Build history of the part. All positions in model axes, mm. A direction names the side the tool comes from. Round coordinates to 2 decimals unless told otherwise and drop trailing zeros. Write each loop counter-clockwise with the first axis right and the second up, starting at its lowest first coordinate (ties: lowest second). Pieces come first, ordered by that corner, then holes. Notation, with made-up numbers: M 25.25,32.5 L 69.25,32.5 A6 ccw 69.25,36.5 Z; hole C 59,84 d9. An arc over 180 degrees is marked long. Write item = value, one per line.
from build123d import *

# Parameters (mm, degrees)
F0_W     = 1016
F0_H     = 381
F1_DEPTH = 1778
F2_T     = -25.4
F3_R     = 31.75
F4_DEPTH = 1016.001


with BuildPart() as f1:
    # F0 (on Front) → F1 (new body)
    with BuildSketch(Plane.XZ):
        with Locations((0, 190.5)):
            Rectangle(F0_W, F0_H)
    extrude(amount=-F1_DEPTH)

    # F2
    f2_openings = [f1.faces().sort_by_distance(p)[0] for p in [
        (0, 889, 381),
    ]]
    offset(amount=F2_T, openings=f2_openings)

    # F3 (on face) → F4 (cut, through all)
    with BuildSketch(Plane.YZ.offset(508)):
        with Locations((254, 127)):
            Circle(F3_R)
        with Locations((1651, 127)):
            Circle(F3_R)
        with Locations((889, 127)):
            Circle(F3_R)
    extrude(amount=-F4_DEPTH, mode=Mode.SUBTRACT)


solid = f1.part
1. Probe probe 1 along X at (y, z) = (187, 207.5); probe 2 along Y at (x, z) = (-273.5, 324); probe 3 along Z at (x, y) = (-489.5, 1651). List the from-to ranges inside material, lowest first.
Responses:
probe_1 = -508 to -482.6, 482.6 to 508
probe_2 = 0 to 25.4, 1752.6 to 1778
probe_3 = 0 to 95.25, 158.75 to 381
2. Flat gauge pins, fed straight in: pin 1 (8 mm diameter, centred on x = -102.5, y = 833, fed in from -Z); pin 2 (6 mm diameter, centred on x = -370, y = 813, fed in from +Z). Where does each tip first touch, or does it go through?
Responses:
pin_1 = 0
pin_2 = 25.4
3. Band-saw the part on B-B (y = 254). List the corners of the cut face in (x, z), plus the area to 3 significant figures.
Responses:
outline = M -508,0 L 508,0 L 508,95.25 L 482.6,95.25 L 482.6,25.4 L -482.6,25.4 L -482.6,95.25 L -508,95.25 Z; M -508,158.75 L -482.6,158.75 L -482.6,381 L -508,381 Z; M 482.6,158.75 L 508,158.75 L 508,381 L 482.6,381 Z
area = 40,600 mm²
4. Band-saw the part on D-D (x = -82). List the corners of the cut face in (y, z), plus the area to 3 significant figures.
Responses:
outline = M 0,0 L 1778,0 L 1778,381 L 1752.6,381 L 1752.6,25.4 L 25.4,25.4 L 25.4,381 L 0,381 Z
area = 63,200 mm²
5. Mould opens along Z. For faces 3 (the face through (-7, 877, 0)), 4 (the face through (-7, 1778, 193)), 5 (the face through (-7, 877, 25.4)), 6 (the face through (-495.122, 228.804, 107.681)) say: pulls with the +Z half, pulls with the -Z half, needs draft (parallel to the pull), parting line crosses it, or undercut.
Responses:
face_3 = pulls with the -Z half
face_4 = needs draft
face_5 = pulls with the +Z half
face_6 = undercut
6. Band-saw the part on A-A (z = 127). Count the separate pieces of the cut face and the enclosed holes in it, plus the area to 3 significant figures.
Responses:
separate_pieces = 6
enclosed_holes = 0
area = 130,000 mm²
7. Band-saw the part on C-C (z = 326). List the corners of the cut face in (x, y), plus the area to 3 significant figures.
Responses:
outline = M -508,0 L 508,0 L 508,1778 L -508,1778 Z; hole M -482.6,25.4 L 482.6,25.4 L 482.6,1752.6 L -482.6,1752.6 Z
area = 139,000 mm²
8. Tool access for faces 1 (the face through (-7, 25.4, 206)), 2 (the face through (495.48, 1680.33, 114.84)): list every direction of +Z, -Z, +X, -X, +Y, -Y with a clear straight run to the whole face (end or side of a thin tool).
Responses:
face_1 = +Z
face_2 = +X, -X
